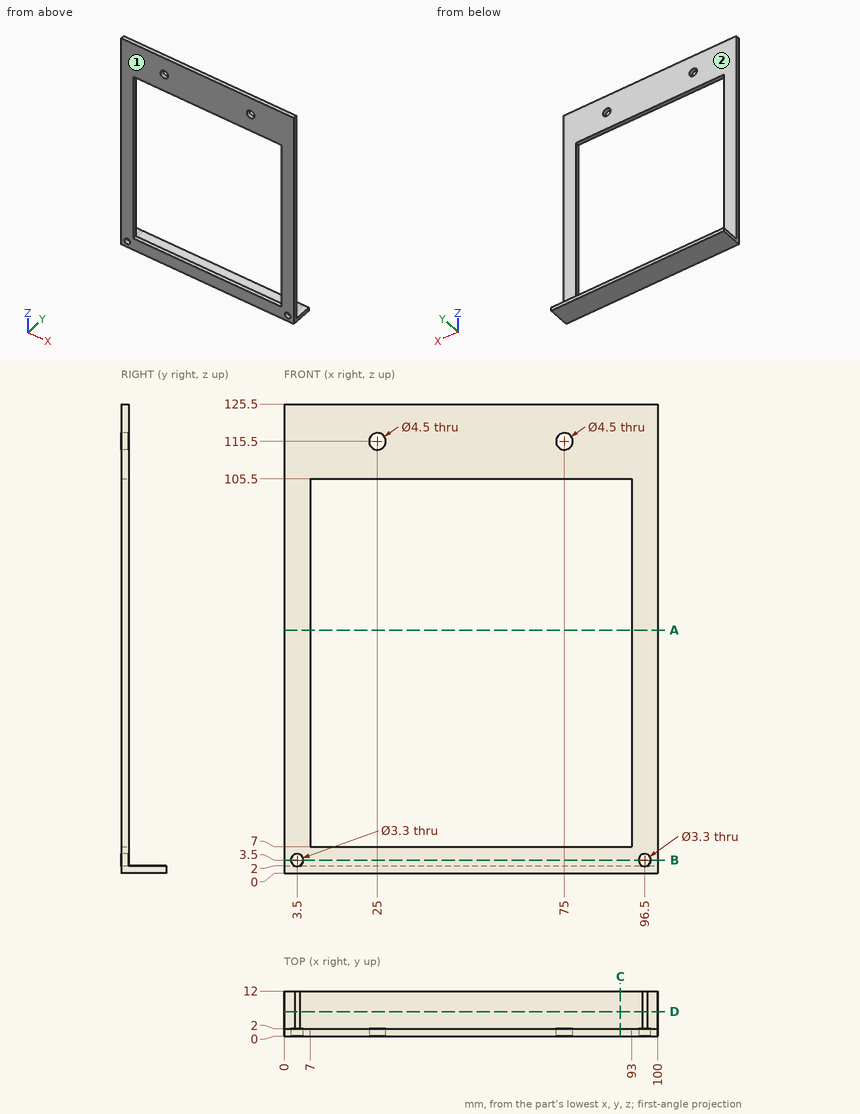
Geometry check sheet. Reference: drawing and pictorial views, mm from the part's lowest x, y, z. A direction names the side the tool comes from. Give positions to 0.01 mm unless a question says otherwise; leave off trailing zeros. Write each loop counter-clockwise with the first axis right and the second up, starting at its lowest first coordinate (ties: lowest second). Pieces come first, ordered by that corner, then holes.
Item 1: Cross-section at C-C (x = 90). Enter the section's corners in (y, z), and give its area (3 significant figures).
Item 2: Gauge pin test, flat end, axial feed: pin 1 (3 mm diameter, centred on x = 56, y = 6.5, fed in from +Z). Record the tip position at first contact, or that the pin passes through.
Item 3: Access from +Z, -Z, +X, -X, +Y, -Y to the whole of each face (thin tool, end or side, straight path). Record for the marked faces 1 and 2.
Item 4: Scan lines: L1, parallel to Z at x = 75, y = 1.4; L2, parallel to X at y = 0.55, z = 115.5; L3, parallel to Y at x = 95, z = 65. Record each from-to range of solid material in increasing order.
Item 5: Cross-section at B-B (z = 3.5). Enter the section's corners in (x, y).
Item 6: Cross-section at A-A (z = 65). Enter the section's corners in (x, y), and give its area (3 significant figures).
Item 7: Cross-section at D-D (y = 6.5). Enter the section's corners in (x, z), and give its area (3 significant figures).
Report:
1. outline: (0, 0) - (12, 0) - (12, 2) - (2, 2) - (2, 7) - (0, 7) - close; (0, 105.5) - (2, 105.5) - (2, 125.5) - (0, 125.5) - close
1. area: 74.0 mm2
2. pin 1: stops at z = 2
3. face 1: +Z, -Z, +X, -X, -Y
3. face 2: +Z, +X, -X, +Y
4. L1: z = 0 to 7, 105.5 to 113.25, 117.75 to 125.5
4. L2: x = 0 to 22.75, 27.25 to 72.75, 77.25 to 100
4. L3: y = 0 to 2
5. outline: (0, 0) - (1.85, 0) - (1.85, 2) - (0, 2) - close; (5.15, 0) - (94.85, 0) - (94.85, 2) - (5.15, 2) - close; (98.15, 0) - (100, 0) - (100, 2) - (98.15, 2) - close
6. outline: (0, 0) - (7, 0) - (7, 2) - (0, 2) - close; (93, 0) - (100, 0) - (100, 2) - (93, 2) - close
6. area: 28.0 mm2
7. outline: (0, 0) - (100, 0) - (100, 2) - (97.19, 2) arc R1.65 cw to (95.81, 2) - (4.19, 2) arc R1.65 cw to (2.81, 2) - (0, 2) - close
7. area: 200 mm2
